Build history of the part. All positions in model axes, mm. A direction names the side the tool comes from. Give positions to 0.01 mm unless a question says otherwise; leave off trailing zeros. Order: outer loops, then holes, each group sorted by start corner. A loop starts at its lowest first (then second) coordinate and runs counter-clockwise, first axis right, second up. Notation, with made-up numbers: M -37.75,58.5 L 9.25,58.5 A10 ccw 9.25,64.5 Z; hole C 33.25,-36 d11. An arc over 180 degrees is marked long. One line per item, written item: value.
Autodesk Inventor part; units mm, degrees
ref_plane "YZ Plane" through (0, 0, 0) normal (1, 0, 0) x (0, 1, 0)
ref_plane "XZ Plane" through (0, 0, 0) normal (0, 1, 0) x (-1, 0, 0)
ref_plane "XY Plane" through (0, 0, 0) normal (0, 0, 1) x (1, 0, 0)
sketch "Sketch1" plane through (0, 0, 0) normal (0, 1, 0) x (-1, 0, 0)
  line L0 (0, 0) -> (79.5, 0)
  line L1 (79.5, 0) -> (79.5, -106)
  line L2 (79.5, -106) -> (0, -106)
  line L3 (0, -106) -> (0, 0)
  dimension "d6" = 106
  dimension "d7" = 79.5
extrude "Extrusion1" add sketch "Sketch1" along normal blind 2
sketch "Sketch2" plane through (0, 0, 0) normal (0, -1, 0) x (1, 0, 0)
  line L0 (0, -106) -> (-79.5, -106)
  line L1 (0, 0) -> (0, -106)
  line L2 (-79.5, 0) -> (0, 0)
  line L3 (-79.5, -106) -> (-79.5, 0)
  line L4 (-3, -103) -> (-6, -103)
  line L5 (-6, -103) -> (-6, -96)
  line L6 (-6, -96) -> (-3, -96)
  line L7 (-3, -96) -> (-3, -103)
  dimension "d10" = 7
  dimension "d11" = 3
  dimension "d12" = 3
  dimension "d13" = 3
extrude "Extrusion2" add sketch "Sketch2" along normal blind 48 contours L4 L5 L6 L7
sketch "Sketch3" plane through (-3, 0, -96) normal (1, 0, 0) x (0, 0, -1)
  circle A0 centre (3.5, -43) radius 1.5
  line L0 (7, -48) -> (0, -48)
  line L1 (7, 0) -> (7, -48)
  point P0 (-96, 0)
  dimension "d14" = 5
  dimension "d16" = 3
  dimension "d22" = 3.5
extrude "Extrusion3" cut sketch "Sketch3" against normal blind 33
sketch "Sketch4" plane through (-3, 0, -96) normal (1, 0, 0) x (0, 0, -1)
  circle A0 centre (3.5, -43) radius 1.5
  line L0 (0, 0) -> (7, 0)
  line L1 (0, 0) -> (0, -48)
  line L2 (7, -48) -> (0, -48)
  line L3 (7, 0) -> (7, -48)
  line L4 (0, -48) -> (7, -48)
  line L5 (7, -48) -> (7, -47)
  line L6 (7, -47) -> (0, -47)
  line L7 (0, -47) -> (0, -48)
  point P0 (-96, 0)
  point P1 (0, -47)
  dimension "d19" = 1
extrude "Extrusion4" cut sketch "Sketch4" against normal blind 33 contours L6 L3 L2 L1
properties part number "Enclosure Lid"
1) Saw through at C-C, the plane z = -82. Write the cut outline in (x, y), then the cut area to 3 significant figures.
Check values:
outline: M -79.5,0 L 0,0 L 0,2 L -79.5,2 Z
area: 159 mm^2
2) Saw through at B-B, the plane y = -43. Write the cut outline in (x, z).
Check values:
outline: M -6,-103 L -3,-103 L -3,-101 L -6,-101 Z; M -6,-98 L -3,-98 L -3,-96 L -6,-96 Z
3) Tool access for faces 1 (the face through (-3, -23, -99)), 2 (the face through (-39, 2, -52)): list every direction of +Z, -Z, +X, -X, +Y, -Y with a clear straight run to the whole face (end or side of a thin tool).
Check values:
face 1: +Z, -Z, +X, -Y
face 2: +Z, -Z, +X, -X, +Y
4) Saw through at D-D, the plane x = -11. Write the cut outline in (y, z).
Check values:
outline: M 0,-106 L 2,-106 L 2,0 L 0,0 Z
5) Mould opens along Z. For faces 3 (the face through (-4.48, -44.33, -100.19)), 4 (the face through (-6, -23, -100)), 5 (the face through (-4, -23, -103)), 6 (the face through (-5, -23, -96)) say: released by +Z, released by -Z, zero draft, split by the parting line, or undercut.
Check values:
face 3: undercut
face 4: zero draft
face 5: released by -Z
face 6: released by +Z
6) Saw through at A-A, the plane z = -99.5. Write the cut outline in (x, y), then the cut area to 3 significant figures.
Check values:
outline: M -79.5,0 L -6,0 L -6,-41.5 L -3,-41.5 L -3,0 L 0,0 L 0,2 L -79.5,2 Z; M -6,-47 L -3,-47 L -3,-44.5 L -6,-44.5 Z
area: 291 mm^2
7) Drill centre lines: probe 1 along Y at (x, z) = (-3.65, -99.5); probe 2 along Y at (x, z) = (-43.5, -40); probe 3 along X at (y, z) = (-41, -100.5). Where is each one in solid material? Low to high. Write a range as from..to.
Check values:
probe 1: -47..-44.5, -41.5..2
probe 2: 0..2
probe 3: -6..-3
8) Pin check, flat tips, straight feed: pin 1 (1.5 mm diameter, centred on x = -5, y = -15, fed in from -Z); pin 2 (5.5 mm diameter, centred on y = -14.5, z = -101, fed in from -X); pin 3 (1.5 mm diameter, centred on x = -54.5, z = -74.5, fed in from -Y). Stop position of each tip, or through.
Check values:
pin 1: z = -103
pin 2: x = -6
pin 3: y = 0
